Drawing for the job (mm, zero at the part's lowest x, y, z). A direction names the side the tool comes from. Give positions to 0.01 mm unless a question says otherwise; leave off trailing zeros. Order: outer loops, then holes, each group sorted by start corner. A loop starts at its lowest first (then second) coordinate and runs counter-clockwise, first axis right, second up. Notation, with made-up numbers: (-17, 27.5) -> (12, 27.5) arc R19 ccw to (12, 33.5) -> close; hole circle Ø8 at (-33, -39.5). An arc over 180 degrees is marked (long way). Use one line per item in the form item = value. Start each with the question number.
1) Tool access for the marked faces 1, 2 and 3: list every direction of +Z, -Z, +X, -X, +Y, -Y with a clear straight run to the whole face (end or side of a thin tool).
2) Probe line 1 (Y direction, x = 54.5, z = 4.75) (1 decimal); line 2 (X direction, y = 39.5, z = 5.5) (1 decimal); line 3 (Y direction, x = 71, z = 6.75) (1 decimal). List the from-to ranges inside material, lowest first.
3) Cut at D-D, the plane y = 59. Give the cut face in (x, z).
4) Cut at C-C, the plane x = 6. Give the cut face in (y, z), and give its area (3 significant figures).
5) Cut at B-B, the plane x = 54.15. State how many separate pieces and enclosed holes the cut face has.
6) Cut at A-A, the plane y = 38.1. Give the cut face in (x, z).
7) Drop flat-ended pins along their axis: P1, Ø1.5, axis at x = 37.5, y = 13, coming from the +Z side; P2, Ø1.5, axis at x = 64, z = 2, coming from the -Y side; P3, Ø3, axis at y = 54, z = 8.5, coming from the +X side (1 decimal). Give the stop position or say it passes through.
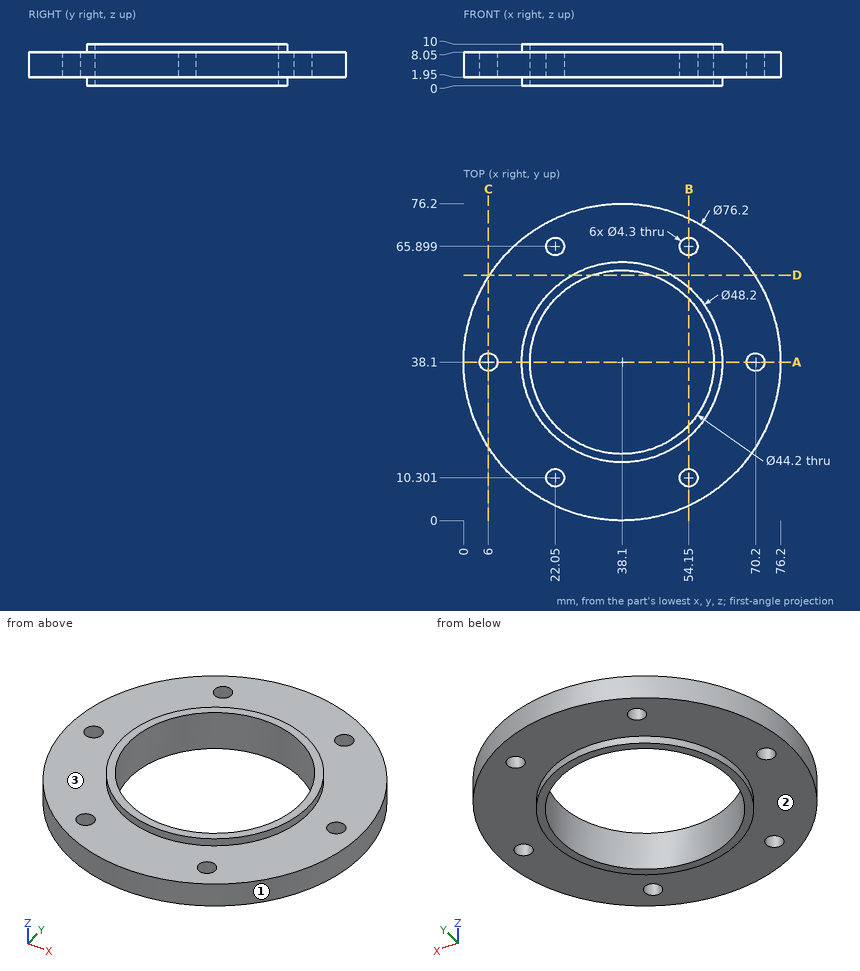
Result:
q1.face_1 = +Z, -Z
q1.face_2 = -Z
q1.face_3 = +Z
q2.line_1 = 3.7 to 8.2, 12.4 to 23.3, 52.9 to 63.8, 68 to 72.5
q2.line_2 = 0 to 4.4, 7.6 to 16, 60.2 to 68.6, 71.8 to 76.2
q2.line_3 = 18.9 to 36.1, 40.1 to 57.3
q3.outline = (6.24, 1.95) -> (26.1, 1.95) -> (26.1, 0) -> (30.92, 0) -> (30.92, 10) -> (26.1, 10) -> (26.1, 8.05) -> (6.24, 8.05) -> close; (45.28, 0) -> (50.1, 0) -> (50.1, 1.95) -> (69.96, 1.95) -> (69.96, 8.05) -> (50.1, 8.05) -> (50.1, 10) -> (45.28, 10) -> close
q4.outline = (17.58, 1.95) -> (35.95, 1.95) -> (35.95, 8.05) -> (17.58, 8.05) -> close; (40.25, 1.95) -> (58.62, 1.95) -> (58.62, 8.05) -> (40.25, 8.05) -> close
q4.area = 224 mm²
q5.separate_pieces = 4
q5.enclosed_holes = 0
q6.outline = (0, 1.95) -> (3.85, 1.95) -> (3.85, 8.05) -> (0, 8.05) -> close; (8.15, 1.95) -> (14, 1.95) -> (14, 0) -> (16, 0) -> (16, 10) -> (14, 10) -> (14, 8.05) -> (8.15, 8.05) -> close; (60.2, 0) -> (62.2, 0) -> (62.2, 1.95) -> (68.05, 1.95) -> (68.05, 8.05) -> (62.2, 8.05) -> (62.2, 10) -> (60.2, 10) -> close; (72.35, 1.95) -> (76.2, 1.95) -> (76.2, 8.05) -> (72.35, 8.05) -> close
q7.P1 = 8.05
q7.P2 = 9.48
q7.P3 = 73.3
